from build123d import *

# Parameters (mm, degrees)
F1_DEPTH = 10
F2_DEPTH = 7
F0_W     = 12.2951196297
F0_H     = 10
F3_DEPTH = 5


with BuildPart() as f1:
    # F0 (on Front) → F1 (new body)
    with BuildSketch(Plane.XZ):
        with BuildLine():
            ThreePointArc((27.7048803703, -28.3328760415), (25.5461182747, -15.3698241684), (19.3028446771, -3.8059795467))
            ThreePointArc((19.3028446771, -3.8059795467), (15.9891516178, -0.0486047941), (12.2317768652, 3.2650882652))
            ThreePointArc((12.2317768652, 3.2650882652), (0.6679322435, 9.5083618628), (-12.2951196297, 11.6671239585))
            ThreePointArc((-12.2951196297, 11.6671239585), (-25.2581715028, 9.5083618628), (-36.8220161245, 3.2650882652))
            ThreePointArc((-36.8220161245, 3.2650882652), (-40.5793860243, -0.0485999413), (-43.8930755201, -3.805968704))
            ThreePointArc((-43.8930755201, -3.805968704), (-52.2951196297, -28.3328691786), (-43.8930839364, -52.8597725364))
            ThreePointArc((-43.8930839364, -52.8597725364), (-40.5793908771, -56.617147289), (-36.8220161245, -59.9308403483))
            ThreePointArc((-36.8220161245, -59.9308403483), (-12.2951196297, -68.3328760415), (12.2317768652, -59.9308403483))
            ThreePointArc((12.2317768652, -59.9308403483), (15.9891516178, -56.617147289), (19.3028446771, -52.8597725364))
            ThreePointArc((19.3028446771, -52.8597725364), (25.5461182747, -41.2959279147), (27.7048803703, -28.3328760415))
        make_face()
    extrude(amount=F1_DEPTH)

    # F0 (on Front) → F2 (join)
    with BuildSketch(Plane.XZ):
        with BuildLine():
            ThreePointArc((-43.8930755201, -3.805968704), (-40.5793860243, -0.0485999413), (-36.8220161245, 3.2650882652))
            Line((-36.8220161245, 3.2650882652), (-40.6279956712, 7.0710678119))
            Line((-40.6279956712, 7.0710678119), (-44.1635295771, 3.5355339059))
            Line((-44.1635295771, 3.5355339059), (-47.6990634831, 0))
            Line((-47.6990634831, 0), (-44.1635295771, -3.5355339059))
            Line((-44.1635295771, -3.5355339059), (-43.8930755201, -3.805968704))
        make_face()
        Polygon((-57.7240518178, 24.1671239585), (-67.7240518178, 34.1671239585), (-74.7951196297, 34.1671239585), (-74.7951196297, 27.0960561466), (-64.7951196297, 17.0960561466), (-47.6990634831, 0), (-44.1635295771, 3.5355339059), (-40.6279956712, 7.0710678119), align=None)
        Polygon((-74.7951196297, -90.8328760415), (-67.7240518178, -90.8328760415), (-57.7240518178, -80.8328760415), (-40.6279956712, -63.7368198949), (-44.1635295771, -60.201285989), (-47.6990634831, -56.6657520831), (-64.7951196297, -73.7618082297), (-74.7951196297, -83.7618082297), align=None)
        with BuildLine():
            Line((-40.6279956712, -63.7368198949), (-36.8220161245, -59.9308403483))
            ThreePointArc((-36.8220161245, -59.9308403483), (-40.5793908771, -56.617147289), (-43.8930839364, -52.8597725364))
            Line((-43.8930839364, -52.8597725364), (-47.6990634831, -56.6657520831))
            Line((-47.6990634831, -56.6657520831), (-44.1635295771, -60.201285989))
            Line((-44.1635295771, -60.201285989), (-40.6279956712, -63.7368198949))
        make_face()
        Polygon((40.2048803703, 17.0960561466), (50.2048803703, 27.0960561466), (50.2048803703, 34.1671239585), (43.1338125585, 34.1671239585), (33.1338125585, 24.1671239585), (24.2192459165, 15.2525573165), (27.7547798224, 11.7170234106), (31.2903137284, 8.1814895046), align=None)
        with BuildLine():
            Line((19.3028446771, -3.8059795467), (31.2903137284, 8.1814895046))
            Line((31.2903137284, 8.1814895046), (27.7547798224, 11.7170234106))
            Line((27.7547798224, 11.7170234106), (24.2192459165, 15.2525573165))
            Line((24.2192459165, 15.2525573165), (12.2317768652, 3.2650882652))
            ThreePointArc((12.2317768652, 3.2650882652), (15.9891516178, -0.0486047941), (19.3028446771, -3.8059795467))
        make_face()
        Polygon((50.2048803703, -90.8328760415), (50.2048803703, -83.7618082297), (40.2048803703, -73.7618082297), (32.423708156, -65.9806360153), (28.88817425, -69.5161699212), (25.3526403441, -73.0517038272), (33.1338125585, -80.8328760415), (43.1338125585, -90.8328760415), align=None)
        with BuildLine():
            Line((28.88817425, -69.5161699212), (32.423708156, -65.9806360153))
            Line((32.423708156, -65.9806360153), (19.3028446771, -52.8597725364))
            ThreePointArc((19.3028446771, -52.8597725364), (15.9891516178, -56.617147289), (12.2317768652, -59.9308403483))
            Line((12.2317768652, -59.9308403483), (25.3526403441, -73.0517038272))
            Line((25.3526403441, -73.0517038272), (28.88817425, -69.5161699212))
        make_face()
    extrude(amount=F2_DEPTH)

    # F0 (on Front) → F3 (join)
    with BuildSketch(Plane.XZ):
        Polygon((50.2048803703, -83.7618082297), (50.2048803703, 0), (40.2048803703, 0), (40.2048803703, -73.7618082297), align=None)
        Polygon((50.2048803703, 0), (50.2048803703, 9.1671239585), (50.2048803703, 27.0960561466), (40.2048803703, 17.0960561466), (40.2048803703, 0), align=None)
        Polygon((33.1338125585, 24.1671239585), (43.1338125585, 34.1671239585), (0, 34.1671239585), (0, 24.1671239585), align=None)
        with Locations((-6.1475598148, 29.1671239585)):
            Rectangle(F0_W, F0_H)
        Polygon((-12.2951196297, 24.1671239585), (-12.2951196297, 34.1671239585), (-67.7240518178, 34.1671239585), (-57.7240518178, 24.1671239585), align=None)
        Polygon((-64.7951196297, 17.0960561466), (-74.7951196297, 27.0960561466), (-74.7951196297, -28.3328760415), (-64.7951196297, -28.3328760415), align=None)
        Polygon((-74.7951196297, -28.3328760415), (-74.7951196297, -83.7618082297), (-64.7951196297, -73.7618082297), (-64.7951196297, -28.3328760415), align=None)
        Polygon((-67.7240518178, -90.8328760415), (0, -90.8328760415), (0, -80.8328760415), (-57.7240518178, -80.8328760415), align=None)
        Polygon((0, -90.8328760415), (43.1338125585, -90.8328760415), (33.1338125585, -80.8328760415), (0, -80.8328760415), align=None)
    extrude(amount=F3_DEPTH)


solid = f1.part
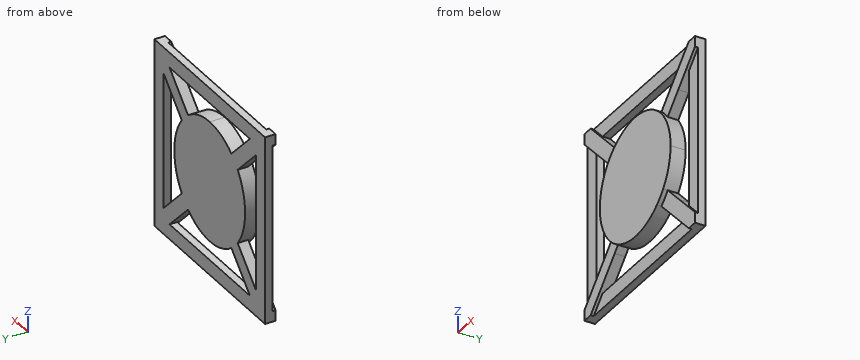
Here's how the part is built. I have some questions about the finished solid (model axes, mm). Coordinates: 2 decimals unless noted, no trailing zeros. Order: outer loops, then holes, each group sorted by start corner. A loop starts at its lowest first (then second) coordinate and runs counter-clockwise, first axis right, second up.
Item 1: If we section it at B-B on x = 23: List the corners of the cut face in (y, z) for me.
Result sheet:
outline: (-10, -47.15) - (0, -47.15) - (0, -9.51) - (-10, -9.51) - close; (-7, -70.7) - (0, -70.7) - (0, -56.56) - (-7, -56.56) - close; (-7, -0.11) - (0, -0.11) - (0, 14.03) - (-7, 14.03) - close; (-5, -90.83) - (0, -90.83) - (0, -80.83) - (-5, -80.83) - close; (-5, 24.17) - (0, 24.17) - (0, 34.17) - (-5, 34.17) - close
Item 2: For P1, Ø19, axis at x = 29, z = 14, coming from the -Y side; P2, Ø3, axis at x = -70, z = -34.5, coming from the -Y side, each with a flat end and sliding along its axis, tell me the tip position at first contact or that it passes through.
Result sheet:
P1: stops at y = -7
P2: stops at y = -5
Item 3: If we section it at D-D on x = 37: List the corners of the cut face in (y, z) for me.
Result sheet:
outline: (-7, -84.7) - (-5, -84.7) - (-5, -90.83) - (0, -90.83) - (0, -70.56) - (-7, -70.56) - close; (-7, 13.89) - (0, 13.89) - (0, 34.17) - (-5, 34.17) - (-5, 28.03) - (-7, 28.03) - close
Item 4: If we section it at C-C on z = -40.5: List the corners of the cut face in (x, y) for me.
Result sheet:
outline: (-74.8, -5) - (-64.8, -5) - (-64.8, 0) - (-74.8, 0) - close; (-50.4, -10) - (25.81, -10) - (25.81, 0) - (-50.4, 0) - close; (40.2, -5) - (50.2, -5) - (50.2, 0) - (40.2, 0) - close
Item 5: If we section it at A-A on y = -3.5: List the corners of the cut face in (x, z) for me, plus the area to 3 significant figures.
Result sheet:
outline: (-74.8, -90.83) - (50.2, -90.83) - (50.2, 34.17) - (-74.8, 34.17) - close; hole (-64.8, -73.76) - (-43.89, -52.86) arc R40 cw to (-43.89, -3.81) - (-44.16, -3.54) - (-64.8, 17.1) - close; hole (-57.72, -80.83) - (33.13, -80.83) - (12.23, -59.93) arc R40 cw to (-36.82, -59.93) - close; hole (-57.72, 24.17) - (-36.82, 3.27) arc R40 cw to (12.23, 3.27) - (33.13, 24.17) - close; hole (19.3, -52.86) - (40.2, -73.76) - (40.2, 17.1) - (19.3, -3.81) arc R40 cw to start
area: 10,900 mm2
Item 6: I need wall thicknesses on line 1 (X direction, y = -0.5, z = -60); line 2 (Z direction, x = 11.5, y = -4); line 3 (X direction, y = -2, z = -42). Which ranges of each line are inside material? Lowest first, please.
Result sheet:
line 1: x = -74.8 to -64.8, -51.03 to -36.89, -36.73 to 12.14, 12.3 to 26.44, 40.2 to 50.2
line 2: z = -90.83 to -80.83, -60.49 to 3.82, 24.17 to 34.17
line 3: x = -74.8 to -64.8, -49.89 to 25.3, 40.2 to 50.2
